```python
from build123d import *
from OCP.BRepFilletAPI import BRepFilletAPI_MakeChamfer

# Parameters (mm, degrees)
ESQUISSE1_W                  = 125
ESQUISSE1_H                  = 420
BOSS_EXTRU_1_DEPTH           = 15
ENL_V_MAT_EXTRU_1_DEPTH      = 439.463225368
ENL_V_MAT_EXTRU_1_DEPTH_BACK = 439.463225368
ESQUISSE2_R                  = 15
CHANFREIN1_SIZE              = 12
CHANFREIN1_SIZE2             = 6.92820323
ESQUISSE3_W                  = 60
ESQUISSE3_H                  = 29
BOSS_EXTRU_2_DEPTH           = 15
CONG_1_R                     = 20
ENL_V_MAT_EXTRU_2_DEPTH      = 467.316416181
ENL_V_MAT_EXTRU_2_DEPTH_BACK = 467.316416181
ESQUISSE4_R                  = 1.65
ESQUISSE5_W                  = 10
ESQUISSE5_H                  = 400
BOSS_EXTRU_3_DEPTH           = 15


with BuildPart() as part:
    # Esquisse1 → Boss.-Extru.1 (new body)
    with BuildSketch(Plane.XY):
        with Locations((62.5, 210)):
            Rectangle(ESQUISSE1_W, ESQUISSE1_H)
    extrude(amount=BOSS_EXTRU_1_DEPTH)

    # Esquisse2 → Enlèv. mat.-Extru.1 (cut, two sides: drawn at the far end of the back side and taken through both)
    with BuildSketch(Plane.XY.offset(15).offset(-ENL_V_MAT_EXTRU_1_DEPTH_BACK)):
        with Locations((28.75, 245.5)):
            Circle(ESQUISSE2_R)
        with Locations(Location((99.25, 245.5, 0), (0, 0, 180))):
            Circle(ESQUISSE2_R)
        with Locations((99.25, 174.5)):
            Circle(ESQUISSE2_R)
        with Locations(Location((28.75, 174.5, 0), (0, 0, 180))):
            Circle(ESQUISSE2_R)
        with Locations((28.75, 103.5)):
            Circle(ESQUISSE2_R)
        with Locations(Location((99.25, 103.5, 0), (0, 0, 180))):
            Circle(ESQUISSE2_R)
        with Locations((99.25, 32.5)):
            Circle(ESQUISSE2_R)
        with Locations(Location((28.75, 32.5, 0), (0, 0, 180))):
            Circle(ESQUISSE2_R)
        with Locations((28.75, 387.5)):
            Circle(ESQUISSE2_R)
        with Locations(Location((99.25, 387.5, 0), (0, 0, 180))):
            Circle(ESQUISSE2_R)
        with Locations((99.25, 316.5)):
            Circle(ESQUISSE2_R)
        with Locations(Location((28.75, 316.5, 0), (0, 0, 180))):
            Circle(ESQUISSE2_R)
    extrude(amount=ENL_V_MAT_EXTRU_1_DEPTH + ENL_V_MAT_EXTRU_1_DEPTH_BACK, mode=Mode.SUBTRACT)

    # Chanfrein1: one chamfer whose edges measure the first distance from different faces: ONE call of the kernel's chamfer builder (chamfer() names one face for all edges)
    chanfrein1_edges_1 = [part.edges().sort_by_distance(p)[0] for p in [
        (13.75, 245.5, 0),
    ]]
    chanfrein1_side_1 = [part.faces().sort_by_distance(p)[0] for p in [
        (13.75, 245.5, 7.5),
    ]]
    chanfrein1_edges_2 = [part.edges().sort_by_distance(p)[0] for p in [
        (84.25, 32.5, 0),
    ]]
    chanfrein1_side_2 = [part.faces().sort_by_distance(p)[0] for p in [
        (84.25, 32.5, 7.5),
    ]]
    chanfrein1_edges_3 = [part.edges().sort_by_distance(p)[0] for p in [
        (43.75, 32.5, 0),
    ]]
    chanfrein1_side_3 = [part.faces().sort_by_distance(p)[0] for p in [
        (43.75, 32.5, 7.5),
    ]]
    chanfrein1_edges_4 = [part.edges().sort_by_distance(p)[0] for p in [
        (13.75, 387.5, 0),
    ]]
    chanfrein1_side_4 = [part.faces().sort_by_distance(p)[0] for p in [
        (13.75, 387.5, 7.5),
    ]]
    chanfrein1_edges_5 = [part.edges().sort_by_distance(p)[0] for p in [
        (114.25, 387.5, 0),
    ]]
    chanfrein1_side_5 = [part.faces().sort_by_distance(p)[0] for p in [
        (114.25, 387.5, 7.5),
    ]]
    chanfrein1_edges_6 = [part.edges().sort_by_distance(p)[0] for p in [
        (84.25, 316.5, 0),
    ]]
    chanfrein1_side_6 = [part.faces().sort_by_distance(p)[0] for p in [
        (84.25, 316.5, 7.5),
    ]]
    chanfrein1_edges_7 = [part.edges().sort_by_distance(p)[0] for p in [
        (43.75, 316.5, 0),
    ]]
    chanfrein1_side_7 = [part.faces().sort_by_distance(p)[0] for p in [
        (43.75, 316.5, 7.5),
    ]]
    chanfrein1_edges_8 = [part.edges().sort_by_distance(p)[0] for p in [
        (114.25, 245.5, 0),
    ]]
    chanfrein1_side_8 = [part.faces().sort_by_distance(p)[0] for p in [
        (114.25, 245.5, 7.5),
    ]]
    chanfrein1_edges_9 = [part.edges().sort_by_distance(p)[0] for p in [
        (84.25, 174.5, 0),
    ]]
    chanfrein1_side_9 = [part.faces().sort_by_distance(p)[0] for p in [
        (84.25, 174.5, 7.5),
    ]]
    chanfrein1_edges_10 = [part.edges().sort_by_distance(p)[0] for p in [
        (43.75, 174.5, 0),
    ]]
    chanfrein1_side_10 = [part.faces().sort_by_distance(p)[0] for p in [
        (43.75, 174.5, 7.5),
    ]]
    chanfrein1_edges_11 = [part.edges().sort_by_distance(p)[0] for p in [
        (13.75, 103.5, 0),
    ]]
    chanfrein1_side_11 = [part.faces().sort_by_distance(p)[0] for p in [
        (13.75, 103.5, 7.5),
    ]]
    chanfrein1_edges_12 = [part.edges().sort_by_distance(p)[0] for p in [
        (114.25, 103.5, 0),
    ]]
    chanfrein1_side_12 = [part.faces().sort_by_distance(p)[0] for p in [
        (114.25, 103.5, 7.5),
    ]]
    chanfrein1 = BRepFilletAPI_MakeChamfer(part.part.solid().wrapped)
    for e in chanfrein1_edges_1:
        chanfrein1.Add(CHANFREIN1_SIZE, CHANFREIN1_SIZE2, e.wrapped, chanfrein1_side_1[0].wrapped)  # the first distance lies on this face
    for e in chanfrein1_edges_2:
        chanfrein1.Add(CHANFREIN1_SIZE, CHANFREIN1_SIZE2, e.wrapped, chanfrein1_side_2[0].wrapped)  # the first distance lies on this face
    for e in chanfrein1_edges_3:
        chanfrein1.Add(CHANFREIN1_SIZE, CHANFREIN1_SIZE2, e.wrapped, chanfrein1_side_3[0].wrapped)  # the first distance lies on this face
    for e in chanfrein1_edges_4:
        chanfrein1.Add(CHANFREIN1_SIZE, CHANFREIN1_SIZE2, e.wrapped, chanfrein1_side_4[0].wrapped)  # the first distance lies on this face
    for e in chanfrein1_edges_5:
        chanfrein1.Add(CHANFREIN1_SIZE, CHANFREIN1_SIZE2, e.wrapped, chanfrein1_side_5[0].wrapped)  # the first distance lies on this face
    for e in chanfrein1_edges_6:
        chanfrein1.Add(CHANFREIN1_SIZE, CHANFREIN1_SIZE2, e.wrapped, chanfrein1_side_6[0].wrapped)  # the first distance lies on this face
    for e in chanfrein1_edges_7:
        chanfrein1.Add(CHANFREIN1_SIZE, CHANFREIN1_SIZE2, e.wrapped, chanfrein1_side_7[0].wrapped)  # the first distance lies on this face
    for e in chanfrein1_edges_8:
        chanfrein1.Add(CHANFREIN1_SIZE, CHANFREIN1_SIZE2, e.wrapped, chanfrein1_side_8[0].wrapped)  # the first distance lies on this face
    for e in chanfrein1_edges_9:
        chanfrein1.Add(CHANFREIN1_SIZE, CHANFREIN1_SIZE2, e.wrapped, chanfrein1_side_9[0].wrapped)  # the first distance lies on this face
    for e in chanfrein1_edges_10:
        chanfrein1.Add(CHANFREIN1_SIZE, CHANFREIN1_SIZE2, e.wrapped, chanfrein1_side_10[0].wrapped)  # the first distance lies on this face
    for e in chanfrein1_edges_11:
        chanfrein1.Add(CHANFREIN1_SIZE, CHANFREIN1_SIZE2, e.wrapped, chanfrein1_side_11[0].wrapped)  # the first distance lies on this face
    for e in chanfrein1_edges_12:
        chanfrein1.Add(CHANFREIN1_SIZE, CHANFREIN1_SIZE2, e.wrapped, chanfrein1_side_12[0].wrapped)  # the first distance lies on this face
    add(Compound.cast(chanfrein1.Shape()), mode=Mode.REPLACE)

    # Esquisse3 → Boss.-Extru.2 (add)
    with BuildSketch(Plane.XY.offset(15)):
        with Locations((95, 434.5)):
            Rectangle(ESQUISSE3_W, ESQUISSE3_H)
        with Locations((95, -14.5)):
            Rectangle(ESQUISSE3_W, ESQUISSE3_H)
    extrude(amount=-BOSS_EXTRU_2_DEPTH)

    # Congé1
    cong_1_edges = [part.edges().sort_by_distance(p)[0] for p in [
        (0, 420, 7.5),
        (0, 0, 7.5),
    ]]
    fillet(cong_1_edges, radius=CONG_1_R)

    # Esquisse4 → Enlèv. mat.-Extru.2 (cut, two sides: drawn at the far end of the back side and taken through both)
    with BuildSketch(Plane.XY.offset(15).offset(-ENL_V_MAT_EXTRU_2_DEPTH_BACK)):
        with Locations(Location((13.75, 405, 0), (0, 0, 356.297009275))):
            Circle(ESQUISSE4_R)
        with Locations((13.75, 275)):
            Circle(ESQUISSE4_R)
        with Locations(Location((43.75, 275, 0), (0, 0, 180))):
            Circle(ESQUISSE4_R)
        with Locations(Location((43.75, 405, 0), (0, 0, 275.094419985))):
            Circle(ESQUISSE4_R)
        with Locations(Location((43.75, 15, 0), (0, 0, 84.905577747))):
            Circle(ESQUISSE4_R)
        with Locations((43.75, 145)):
            Circle(ESQUISSE4_R)
        with Locations(Location((13.75, 145, 0), (0, 0, 180))):
            Circle(ESQUISSE4_R)
        with Locations(Location((13.75, 15, 0), (0, 0, 3.702988457))):
            Circle(ESQUISSE4_R)
    extrude(amount=ENL_V_MAT_EXTRU_2_DEPTH + ENL_V_MAT_EXTRU_2_DEPTH_BACK, mode=Mode.SUBTRACT)

    # Esquisse5 → Boss.-Extru.3 (add)
    with BuildSketch(Plane.XY.offset(15)):
        with Locations((130, 210)):
            Rectangle(ESQUISSE5_W, ESQUISSE5_H)
    extrude(amount=-BOSS_EXTRU_3_DEPTH)


solid = part.part
```
CAD build for the part. Positions are in the model's coordinates, mm. A direction names the side the tool comes from. Round coordinates to 2 decimals unless told otherwise and drop trailing zeros. Order: outer loops, then holes, each group sorted by start corner. A loop starts at its lowest first (then second) coordinate and runs counter-clockwise, first axis right, second up. Notation, with made-up numbers: (63.5, 69.5) -> (95.5, 69.5) arc R22 cw to (95.5, 106.5) -> close; hole circle Ø5 at (27.25, 87). An arc over 180 degrees is marked (long way). Write item = value, one per line.
(1) 3-axis set-ups, long thin cutter, end or side, ignore diameter. For faces 4 (the flat face through (42, 0, 7)), 5 (the cylindrical face through (26.797, 402.372, 13.479)): which of +Z, -Z, +X, -X, +Y, -Y reach the whole face in a straight line?
Answers follow:
face_4 = +Z, -Z, -X, -Y
face_5 = +Z, -Z
(2) Cut at B-B (z = 8.75). State how many separate pieces and enclosed holes the cut face has, plus the area to 3 significant figures.
Answers follow:
separate_pieces = 1
enclosed_holes = 20
area = 49,000 mm²
(3) Drill centre lines: L1, parallel to X at y = 386, z = 13; L2, parallel to X at y = 391, z = 8.5; L3, parallel to X at y = -0.5, z = 12.5. Where is each one in solid material? Low to high.
Answers follow:
L1 = 0 to 13.83, 43.67 to 84.33, 114.17 to 135
L2 = 0 to 12.09, 45.41 to 82.59, 115.91 to 135
L3 = 65 to 125
(4) Cut at A-A (y = 174.5). Write the cut outline in (x, z).
Answers follow:
outline = (0, 0) -> (6.82, 0) -> (13.75, 12) -> (13.75, 15) -> (0, 15) -> close; (43.75, 12) -> (50.68, 0) -> (77.32, 0) -> (84.25, 12) -> (84.25, 15) -> (43.75, 15) -> close; (114.25, 12) -> (121.18, 0) -> (135, 0) -> (135, 15) -> (114.25, 15) -> close
(5) Flat gauge pins, fed straight in: P1, Ø2.5, axis at x = 43.75, y = 405, coming from the +Z side; P2, Ø1, axis at x = 22.5, z = 11, coming from the +Y side; P3, Ø2, axis at x = 58.5, z = 4.5, coming from the -Y side; P4, Ø7.5, axis at y = 426, z = 4, coming from the +X side. Where does each tip first touch, or does it go through?
Answers follow:
P1 = through
P2 = 420
P3 = 0
P4 = 125
(6) Cut at D-D (x = 59). Write the cut outline in (y, z).
Answers follow:
outline = (0, 0) -> (420, 0) -> (420, 15) -> (0, 15) -> close
(7) Pull direction Y, two halves, no side cores. Call faces 1 (the flat face through (130, 10, 8)), 2 (the flat face through (125, -10, 8)), 3 (the conical face through (101.26, 118.8, 11.25)): +Y half, -Y half, draft (parallel to the pull), parting line (faces both ways), or undercut.
Answers follow:
face_1 = -Y half
face_2 = draft
face_3 = undercut
